```python
from build123d import *

# Parameters (mm, degrees)
SKETCH1_W                       = 15
SKETCH1_H                       = 6
MAIN_BODY_EXT_DEPTH             = 9.3
EMISSION_PATH_EXT_DEPTH         = 9
SKETCH3_R                       = 1.25
EMISSION_AND_GRIN_CUT_DEPTH     = 21.003499694
FIBER_FERRULE_CUT_REACH         = 25.851
FIBER_FERRULE_CUT_END_RADIUS    = 1.25
SKETCH4_R                       = 0.675
FIBER_START                     = 3
SKETCH41_R                      = 1.675
SKETCH41_R_2                    = 0.675
FIBER_FERRULE_PORT_EXT_DEPTH    = 3
SKETCH5_W                       = 15
SKETCH5_H                       = 8.3
FILTERSET_CUT1_DEPTH            = 0.9
FILTERSET_CUT2_DEPTH            = 4.2
SKETCH10_R                      = 2.5
EMISSION_LENS_CUT_DEPTH         = 8.5
EXCITATION_PATHWAY_CUT_REACH    = 24.231
SKETCH40_R                      = 1.95
EXCITATION_PATHWAY_CUT_2_DEPTH  = 2.1
SKETCH15_R                      = 0.795
MAGNETS_CUT_DEPTH               = 0.9
SCREW_HOLES_CUT_DEPTH           = 22.705989957
SCREW_HOLES_CUT_DEPTH_BACK      = 3
SKETCH18_R                      = 0.375
EXTERNAL_FILLET_1_R             = 1.5
EMISSION_PATHWAY_CUT_DEPTH      = 15.942891286
EMISSION_PATHWAY_CUT_DEPTH_BACK = 4
SKETCH28_R                      = 1.5
CUT_EXTRUDE16_DEPTH             = 9
CUT_EXTRUDE17_REACH             = 16.673
SKETCH37_R                      = 2
LENS_WALL_THICKNESS_EXT_DEPTH   = 6
BASEPLATE_NOTCH_CUT_DEPTH       = 22.386678096
BASEPLATE_NOTCH_CUT_DEPTH_BACK  = 2


with BuildPart() as part:
    # Sketch1 → Main Body Ext (new body)
    with BuildSketch(Plane(origin=(0, 0, 0), x_dir=(1, 0, 0), z_dir=(0, 1, 0))):
        Rectangle(SKETCH1_W, SKETCH1_H)
    extrude(amount=MAIN_BODY_EXT_DEPTH)

    # Sketch8 → Emission Path Ext (add)
    with BuildSketch(Plane(origin=(0, 9.3, 0), x_dir=(1, 0, 0), z_dir=(0, 1, 0))):
        Polygon((-2.75, 3), (-1.5, 1.75), (-1.5, -3), (-7.5, -3), (-7.5, 3), align=None)
    extrude(amount=EMISSION_PATH_EXT_DEPTH)

    # Sketch3 → Emission and Grin Cut (cut, through all)
    with BuildSketch(Plane.XZ):
        with Locations(Location((-4.5, 0, 0), (0, 0, 270))):
            Circle(SKETCH3_R)
    extrude(amount=-EMISSION_AND_GRIN_CUT_DEPTH, mode=Mode.SUBTRACT)

    # Fiber Ferrule Cut: up to this cylinder (the profile starts outside it)
    fiber_ferrule_cut_end = Plane(origin=(-4.5, 4, 0), z_dir=(0, -1, 0)) * Cylinder(FIBER_FERRULE_CUT_END_RADIUS, 55.202, mode=Mode.PRIVATE)
    # Sketch4 → Fiber Ferrule Cut (cut, up to the surface)
    with BuildSketch(Plane(origin=(7.5, 0, 0), x_dir=(0, 0, -1), z_dir=(1, 0, 0)), mode=Mode.PRIVATE) as fiber_ferrule_cut_sk1:
        with Locations((0, 4)):
            Circle(SKETCH4_R)
    fiber_ferrule_cut_tool1 = extrude(fiber_ferrule_cut_sk1.sketch, amount=-FIBER_FERRULE_CUT_REACH, mode=Mode.PRIVATE) - fiber_ferrule_cut_end
    add(fiber_ferrule_cut_tool1.solids().sort_by_distance((7.5, 4, 0))[0], mode=Mode.SUBTRACT)

    # Sketch41 → Fiber Ferrule Port Ext (add)
    with BuildSketch(Plane(origin=(7.5, 0, 0), x_dir=(0, 0, -1), z_dir=(1, 0, 0)).offset(FIBER_START)):
        with Locations(Location((0, 4, 0), (0, 0, 180))):
            Circle(SKETCH41_R)
        with Locations((0, 4)):
            Circle(SKETCH41_R_2, mode=Mode.SUBTRACT)
    extrude(amount=-FIBER_FERRULE_PORT_EXT_DEPTH)

    # Sketch5 → FilterSet Cut1 (cut)
    with BuildSketch(Plane.XY.offset(3)):
        with Locations((0, 5.15)):
            Rectangle(SKETCH5_W, SKETCH5_H)
    extrude(amount=-FILTERSET_CUT1_DEPTH, mode=Mode.SUBTRACT)

    # Sketch6 → FilterSet Cut2 (cut)
    with BuildSketch(Plane.XY.offset(2.1)):
        with BuildLine():
            Line((-2.60588745, 7.591168825), (-6.848528137, 3.348528137))
            ThreePointArc((-6.848528137, 3.348528137), (-6.848528137, 2.5), (-6, 2.5))
            Line((-6, 2.5), (-1.757359313, 6.742640687))
            ThreePointArc((-1.757359313, 6.742640687), (-1.757359313, 7.591168825), (-2.60588745, 7.591168825))
        make_face()
        with BuildLine():
            ThreePointArc((-6.5, 9.3), (-6.782842712, 9.182842712), (-6.9, 8.9))
            Line((-6.9, 8.9), (-6.9, 8.5))
            ThreePointArc((-6.9, 8.5), (-6.782842712, 8.217157288), (-6.5, 8.1))
            Line((-6.5, 8.1), (-2.5, 8.1))
            ThreePointArc((-2.5, 8.1), (-2.217157288, 8.217157288), (-2.1, 8.5))
            Line((-2.1, 8.5), (-2.1, 8.9))
            ThreePointArc((-2.1, 8.9), (-2.217157288, 9.182842712), (-2.5, 9.3))
            Line((-2.5, 9.3), (-6.5, 9.3))
        make_face()
    extrude(amount=-FILTERSET_CUT2_DEPTH, mode=Mode.SUBTRACT)

    # Sketch39 → Excitation Lens Cut (revolve, cut)
    with BuildSketch(Plane.XY, mode=Mode.PRIVATE) as excitation_lens_cut_sk:
        Polygon((0.6, 6.6), (1.88, 6.6), (1.88, 6.9), (3.4, 6.9), (4.81, 6.9), (4.81, 6.35), (6.81, 6.35), (6.81, 4), (4.81, 4), (3.4, 4), (-0.405829172, 4), (-0.9, 4), (-1.76, 4), (-1.76, 6.6), (-0.9, 6.6), align=None)
    revolve(excitation_lens_cut_sk.sketch.rotate(Axis((4.81, 4, 0), (-1, 0, 0)), 90), axis=Axis((4.81, 4, 0), (-1, 0, 0)), mode=Mode.SUBTRACT)

    # Sketch10 → Emission Lens Cut (cut)
    with BuildSketch(Plane(origin=(0, 18.3, 0), x_dir=(1, 0, 0), z_dir=(0, 1, 0))):
        with Locations(Location((-4.5, 0, 0), (0, 0, 270))):
            Circle(SKETCH10_R)
    extrude(amount=-EMISSION_LENS_CUT_DEPTH, mode=Mode.SUBTRACT)

    # Excitation Pathway Cut: up to this plane
    excitation_pathway_cut_end = Plane(origin=(-4.25, 4.25, -10.697056275), z_dir=(-0.7071067811865425, 0.7071067811865526, 0))
    # Sketch40 → Excitation Pathway Cut (cut, up to the surface)
    with BuildSketch(Plane(origin=(-1.76, 0, 0), x_dir=(0, 0, -1), z_dir=(1, 0, 0)), mode=Mode.PRIVATE) as excitation_pathway_cut_sk1:
        with Locations(Location((0, 4, 0), (0, 0, 90))):
            Circle(SKETCH40_R)
    excitation_pathway_cut_tool1 = split(extrude(excitation_pathway_cut_sk1.sketch, amount=-EXCITATION_PATHWAY_CUT_REACH, mode=Mode.PRIVATE), bisect_by=excitation_pathway_cut_end, keep=Keep.BOTH, mode=Mode.PRIVATE)
    add(excitation_pathway_cut_tool1.solids().sort_by_distance((-1.76, 4, 0))[0], mode=Mode.SUBTRACT)

    # Sketch44 → Excitation Pathway Cut 2 (cut)
    with BuildSketch(Plane.XY):
        Polygon((3.4, 1.1), (1.88, 1.1), (1.88, 1.4), (0.6, 1.4), (-0.9, 1.4), (-1.76, 1.4), (-1.76, 6.6), (-0.9, 6.6), (0.6, 6.6), (1.88, 6.6), (1.88, 6.9), (3.4, 6.9), (4.81, 6.9), (4.81, 6.35), (6.81, 6.35), (6.81, 1.65), (4.81, 1.65), (4.81, 1.1), align=None)
    extrude(amount=EXCITATION_PATHWAY_CUT_2_DEPTH, mode=Mode.SUBTRACT)

    # Sketch15 → Magnets Cut (cut)
    with BuildSketch(Plane.XZ):
        with Locations(Location((-6.25, -1.875, 0), (0, 0, 270))):
            Circle(SKETCH15_R)
        with Locations(Location((-6.25, 1.875, 0), (0, 0, 270))):
            Circle(SKETCH15_R)
        with Locations(Location((-1.5, 0, 0), (0, 0, 270))):
            Circle(SKETCH15_R)
    extrude(amount=-MAGNETS_CUT_DEPTH, mode=Mode.SUBTRACT)

    # Sketch18 → Screw Holes Cut (cut, two sides: drawn at the far end of the back side and taken through both)
    with BuildSketch(Plane.XY.offset(2.1).offset(-SCREW_HOLES_CUT_DEPTH_BACK)):
        with Locations(Location((-6.75, 6, 0), (0, 0, 180))):
            Circle(SKETCH18_R)
        with Locations(Location((5.5, 7.5, 0), (0, 0, 180))):
            Circle(SKETCH18_R)
        with Locations(Location((-2.5, 1.51, 0), (0, 0, 180))):
            Circle(SKETCH18_R)
    extrude(amount=SCREW_HOLES_CUT_DEPTH + SCREW_HOLES_CUT_DEPTH_BACK, mode=Mode.SUBTRACT)

    # External Fillet 1
    # the kernel refuses this fillet: 1.5 mm, written as the material it takes off along each edge
    with BuildSketch(Plane(origin=(-7.5, -3.75, -3), x_dir=(1, 0, 0), z_dir=(0, 1, 0))) as external_fillet_1_piece_1:
        with BuildLine():
            CenterArc((EXTERNAL_FILLET_1_R, -EXTERNAL_FILLET_1_R), EXTERNAL_FILLET_1_R, 90, 90)
            Line((0, -EXTERNAL_FILLET_1_R), (0, 0))
            Line((0, 0), (EXTERNAL_FILLET_1_R, 0))
        make_face()
    extrude(amount=25.8, mode=Mode.SUBTRACT)
    with BuildSketch(Plane(origin=(-1.5, 9.3, 3), x_dir=(0, 0, -1), z_dir=(0, 1, 0))) as external_fillet_1_piece_2:
        with BuildLine():
            CenterArc((EXTERNAL_FILLET_1_R, EXTERNAL_FILLET_1_R), EXTERNAL_FILLET_1_R, 180, 90)
            Line((0, EXTERNAL_FILLET_1_R), (0, 0))
            Line((0, 0), (EXTERNAL_FILLET_1_R, 0))
        make_face()
    extrude(amount=12.75, mode=Mode.SUBTRACT)

    # Sketch28 → Emission Pathway Cut (cut, two sides: drawn at the far end of the back side and taken through both)
    with BuildSketch(Plane(origin=(0, 8.1, 0), x_dir=(1, 0, 0), z_dir=(0, 1, 0)).offset(-EMISSION_PATHWAY_CUT_DEPTH_BACK)):
        with Locations(Location((-4.5, 0, 0), (0, 0, 180))):
            Circle(SKETCH28_R)
    extrude(amount=EMISSION_PATHWAY_CUT_DEPTH + EMISSION_PATHWAY_CUT_DEPTH_BACK, mode=Mode.SUBTRACT)

    # Sketch36 → Cut-Extrude16 (cut)
    with BuildSketch(Plane(origin=(0, 18.3, 0), x_dir=(1, 0, 0), z_dir=(0, 1, 0))):
        with BuildLine():
            Line((-7.5, -1.5), (-7.5, -3))
            Line((-7.5, -3), (-6, -3))
            ThreePointArc((-6, -3), (-7.060660172, -2.560660172), (-7.5, -1.5))
        make_face()
    extrude(amount=-CUT_EXTRUDE16_DEPTH, mode=Mode.SUBTRACT)

    # Sketch37 → Cut-Extrude17 (cut, up to next)
    with BuildSketch(Plane(origin=(0, 9.8, 0), x_dir=(1, 0, 0), z_dir=(0, 1, 0)), mode=Mode.PRIVATE) as cut_extrude17_sk1:
        with Locations(Location((-4.5, 0, 0), (0, 0, 180))):
            Circle(SKETCH37_R)
    cut_extrude17_tool1 = extrude(cut_extrude17_sk1.sketch, amount=-CUT_EXTRUDE17_REACH, mode=Mode.PRIVATE) & part.part
    add(cut_extrude17_tool1.solids().sort_by_distance((-4.5, 9.8, 0))[0], mode=Mode.SUBTRACT)

    # Sketch43 → Lens Wall Thickness Ext (add)
    with BuildSketch(Plane.ZY.offset(-5.81)):
        with BuildLine():
            Line((-3, 2.75), (-3, 5.25))
            Line((-3, 5.25), (-3, 5.802775638))
            ThreePointArc((-3, 5.802775638), (-3.5, 4), (-3, 2.197224362))
            Line((-3, 2.197224362), (-3, 2.75))
        make_face()
    extrude(amount=LENS_WALL_THICKNESS_EXT_DEPTH)

    # Sketch45 → Baseplate Notch Cut (cut, two sides: drawn at the far end of the back side and taken through both)
    with BuildSketch(Plane.XZ.offset(-BASEPLATE_NOTCH_CUT_DEPTH_BACK)):
        Polygon((30.47380128, 32.796887648), (7.5, -1.663902268), (6.609270453, -3), (-16.364530827, -37.460789916), (52.557049005, -83.408392475), (99.395381111, -13.150714911), align=None)
    extrude(amount=BASEPLATE_NOTCH_CUT_DEPTH + BASEPLATE_NOTCH_CUT_DEPTH_BACK, mode=Mode.SUBTRACT)


solid = part.part
```
The model under review builds one solid part; all positions refer to its coordinate system, in mm. A direction names the side the tool comes from. Round coordinates to 2 decimals unless told otherwise and drop trailing zeros. Order: outer loops, then holes, each group sorted by start corner. A loop starts at its lowest first (then second) coordinate and runs counter-clockwise, first axis right, second up.
Item 1: Add section C-C, the plane x = 1. State the section outline as (y, z) points.
Working result:
outline: (0, -3) - (2.2, -3) arc R3.5 ccw to (5.8, -3) - (9.3, -3) - (9.3, 2.1) - (6.6, 2.1) - (6.6, 0) arc R2.6 cw to (1.4, 0) - (1.4, 2.1) - (1, 2.1) - (1, 3) - (0, 3) - close
Item 2: Add section A-A, the plane x = -4.5. Count the separate pieces of the cut face and the enclosed holes in it, and give its area (3 significant figures).
Working result:
separate pieces: 4
enclosed holes: 0
area: 27.0 mm2
Item 3: Add section B-B, the plane y = 16.25. State the section outline as (x, z) points.
Working result:
outline: (-7.5, -1.5) arc R1.5 ccw to (-6, -3) - (-2.75, -3) - (-1.5, -1.75) - (-1.5, 1.5) arc R1.5 ccw to (-3, 3) - (-6, 3) arc R1.5 ccw to (-7.5, 1.5) - close; hole circle Ø5 at (-4.5, 0)
Item 4: Draft analysis for pull direction X (two halves, no side actions). For faces 1 (the flat face through (6.81, 3, 0)), 2 (the flat face through (2, 9.3, 0)), 3 (the flat face through (-7.5, 9, 0)), state which applies: released by +X, released by -X, zero draft, split by the parting line, or undercut.
Working result:
face 1: undercut
face 2: zero draft
face 3: released by -X
Item 5: To check wall thickness, follow probe 1 along X at (y, z) = (2.5, 2); probe 2 along Y at (x, z) = (3.5, 2); probe 3 along Y at (x, z) = (7.9, 0) (3 decimals). State the ranges of each line that lie inside material, in increasing order.
Working result:
probe 1: x = -7.5 to -6.85, -6 to -1.76, 6.81 to 7.5
probe 2: y = 0 to 1.1, 6.9 to 9.3
probe 3: y = 2.325 to 3.325, 4.675 to 5.675
Item 6: Machinability: for faces 4 (the flat face through (7.2, 2, -2.6)), 5 (the cylindrical face through (-7.05, 13.86, 2.57)), 6 (the flat face through (7.5, 6, -1)), 7 (the flat face through (0, 6.6, 1)), 8 (the cylindrical face through (-7.026, 0.444, 2.047)), which of the approach directions +Z, -Z, +X, -X, +Y, -Y give a long, thin tool a straight path to every point of the face, cutting with its end or side? Answer none if there is none.
Working result:
face 4: -Z, +X, -Y
face 5: +Z, -X, +Y
face 6: +X
face 7: +Z
face 8: -Y
Item 7: For pin 1 (6.5 mm diameter, centred on x = 2.5, y = 6, fed in from +Z); pin 2 (1.5 mm diameter, centred on x = 1.5, z = 0.5, fed in from +Y), all flat-tipped, find the tip position at first contact; note any pin that passes through.
Working result:
pin 1: stops at z = 2.1
pin 2: stops at y = 9.3
